```python
from build123d import *

# Parameters (mm, degrees)
F0_W     = 254
F0_H     = 203.2
F1_DEPTH = 127
F1_TAPER = 10
F2_W     = 152.4
F2_H     = 101.6
F3_DEPTH = 50.8
F3_TAPER = 20
F4_R     = 5.08


with BuildPart() as f1:
    # F0 (on Top) → F1 (new body)
    with BuildSketch(Plane.XY):
        Rectangle(F0_W, F0_H)
    extrude(amount=F1_DEPTH, taper=F1_TAPER)

    # F2 (on face) → F3 (cut)
    with BuildSketch(Plane.XY.offset(127)):
        with Locations((0, -3.0865822919)):
            Rectangle(F2_W, F2_H)
    extrude(amount=-F3_DEPTH, taper=F3_TAPER, mode=Mode.SUBTRACT)

    # F4
    f4_edges = [f1.edges().sort_by_distance(p)[0] for p in [
        (104.606473, 0, 127),
        (0, -79.206473, 127),
        (0, 79.206473, 127),
        (-104.606473, 0, 127),
        (76.2, -3.086582, 127),
        (0, 47.713418, 127),
        (-76.2, -3.086582, 127),
        (0, -53.886582, 127),
        (-115.803237, 90.403237, 63.5),
        (115.803237, 90.403237, 63.5),
        (115.803237, -90.403237, 63.5),
        (-115.803237, -90.403237, 63.5),
    ]]
    fillet(f4_edges, radius=F4_R)


solid = f1.part
```
Check sheet for the modelled part. Datum: model origin and axes. Units: mm. Round coordinates to 2 decimals unless told otherwise and drop trailing zeros. Write each loop counter-clockwise with the first axis right and the second up, starting at its lowest first coordinate (ties: lowest second). Pieces come first, ordered by that corner, then holes. Notation, with made-up numbers: (-40, 10) -> (-35, 10) arc R4 ccw to (-35, 14) -> close; hole circle Ø4 at (-6, -17). An arc over 180 degrees is marked (long way). One line per question, with ' | ' between items. Start each with the question number.
1. Scan lines: line 1 along Z through (x, y) = (20, -30); line 2 along X through (y, z) = (-21.5, 112); line 3 along X through (y, z) = (20.5, 119.5). Record each from-to range of solid material in increasing order. Write a range as from..to.
2. Release check for a two-part mould opening along Y. For faces 1 (the face through (-2, 1, 0)), 2 (the face through (114.508, -89.185, 62.368)), 3 (the face through (-1, -3, 76.2)), 4 (the face through (-114.585, 89.108, 62.368)) record: +Y half, -Y half, draft (parallel to the pull), parting line (faces both ways), or undercut.
3. Sectioned sample at A-A, the plane x = 92. Record the cut outline in (y, z).
4. Sectioned sample at B-B, the plane y = -63.5. Record the cut outline in (x, z).
5. Depth check by flat-ended pin: pin 1 (10 mm diameter, centred on x = -15, z = 45, fed in from +Y); pin 2 (1.5 mm diameter, centred on y = -1, z = 63.5, fed in from -X); pin 3 (6 mm diameter, centred on x = -22, z = 32, fed in from +Y). Enter the tip coordinate at first touch or a pass-through.
Taken from the geometry:
1) line 1: z = 0..76.2 | line 2: x = -107.25..-70.74, 70.74..107.25 | line 3: x = -105.93..-73.47, 73.47..105.93
2) face 1: draft | face 2: -Y half | face 3: undercut | face 4: +Y half
3) outline: (-101.6, 0) -> (101.6, 0) -> (79.95, 122.8) arc R5.08 ccw to (74.94, 127) -> (-74.94, 127) arc R5.08 ccw to (-79.95, 122.8) -> close
4) outline: (-127, 0) -> (127, 0) -> (105.35, 122.8) arc R5.08 ccw to (100.34, 127) -> (-100.34, 127) arc R5.08 ccw to (-105.35, 122.8) -> close
5) pin 1: stops at y = 94.55 | pin 2: stops at x = -115.94 | pin 3: stops at y = 96.49
